from build123d import *

# Parameters (mm, degrees)
F0_W     = 149.5
F0_H     = 13
F0_R     = 3.1
F1_DEPTH = 18
F3_DEPTH = 10.25
F4_W     = 119.5
F4_H     = 7
F5_DEPTH = 18.001
F7_DEPTH = 25


with BuildPart() as f1:
    # F0 (on Top) → F1 (new body)
    with BuildSketch(Plane.XY):
        Rectangle(F0_W, F0_H)
        with Locations((-68.75, 0.5)):
            Circle(F0_R, mode=Mode.SUBTRACT)
        with Locations((68.75, 0.5)):
            Circle(F0_R, mode=Mode.SUBTRACT)
    extrude(amount=F1_DEPTH)

    # F2 (on Right) → F3 (cut, symmetric)
    with BuildSketch(Plane.YZ):
        Polygon((-6.5, 0), (8.5, 0), (-6.5, 15), align=None)
    extrude(amount=F3_DEPTH, both=True, mode=Mode.SUBTRACT)

    # F4 (on face) → F5 (cut, through all)
    with BuildSketch(Plane.XY.offset(18)):
        with Locations((0, 3)):
            Rectangle(F4_W, F4_H)
    extrude(amount=-F5_DEPTH, mode=Mode.SUBTRACT)

    # F6 (on face) → F7 (cut)
    with BuildSketch(Plane.XZ.offset(6.5)):
        Polygon((-51.359004, 10), (-59.75, 0), (-19.75, 0), (-28.140996, 10), align=None)
        Polygon((28.140996, 10), (19.75, 0), (59.75, 0), (51.359004, 10), align=None)
    extrude(amount=-F7_DEPTH, mode=Mode.SUBTRACT)


solid = f1.part
Geometry check sheet. Reference: the model listing, model coordinates, mm. A direction names the side the tool comes from. Coordinates: 2 decimals unless noted, no trailing zeros. Write each loop counter-clockwise with the first axis right and the second up, starting at its lowest first coordinate (ties: lowest second). Pieces come first, ordered by that corner, then holes. Notation, with made-up numbers: (-37, -37.75) -> (-32, -37.75) arc R36 cw to (-32, -3.75) -> close; hole circle Ø8 at (-12.5, -4.75). An arc over 180 degrees is marked (long way). One line per question, with ' | ' between items.
1. Draft check along X on faces 6 (the flat face through (74.75, 0, 9)), 7 (the flat face through (24.004, -3.542, 5.07)), 8 (the flat face through (-1, -6.5, 17)), 9 (the cylindrical face through (-65.793, 1.431, 8.874)). Enter one of: +X half, -X half, draft (parallel to the pull), parting line (faces both ways), or undercut.
Answers:
face 6: +X half | face 7: undercut | face 8: draft | face 9: undercut
2. Cross-section at D-D on x = 18. Record the cut outline in (y, z).
Answers:
outline: (-6.5, 0) -> (-0.5, 0) -> (-0.5, 18) -> (-6.5, 18) -> close
3. Cross-section at C-C on z = 6.25. Record the cut outline in (x, y), and give its area (3 significant figures).
Answers:
outline: (-74.75, -6.5) -> (-54.51, -6.5) -> (-54.51, -0.5) -> (-59.75, -0.5) -> (-59.75, 6.5) -> (-74.75, 6.5) -> close; (-24.99, -6.5) -> (-10.25, -6.5) -> (-10.25, -0.5) -> (-24.99, -0.5) -> close; (10.25, -6.5) -> (24.99, -6.5) -> (24.99, -0.5) -> (10.25, -0.5) -> close; (54.51, -6.5) -> (74.75, -6.5) -> (74.75, 6.5) -> (59.75, 6.5) -> (59.75, -0.5) -> (54.51, -0.5) -> close; hole circle Ø6.2 at (-68.75, 0.5); hole circle Ø6.2 at (68.75, 0.5) | area: 569 mm²
4. Depth check by flat-ended pin: pin 1 Ø3 at (x, y) = (39.5, -4.5) entering from -Z; pin 2 Ø8 at (x, z) = (-42, 7.5) entering from +Y. Enter the tip coordinate at first touch or a pass-through.
Answers:
pin 1: stops at z = 10 | pin 2: stops at y = -0.5
5. Cross-section at B-B on x = 68.75. Record the cut outline in (y, z), and give its area (3 significant figures).
Answers:
outline: (-6.5, 0) -> (-2.6, 0) -> (-2.6, 18) -> (-6.5, 18) -> close; (3.6, 0) -> (6.5, 0) -> (6.5, 18) -> (3.6, 18) -> close | area: 122 mm²
6. Cross-section at A-A on z = 16.5. Record the cut outline in (x, y).
Answers:
outline: (-74.75, -6.5) -> (74.75, -6.5) -> (74.75, 6.5) -> (59.75, 6.5) -> (59.75, -0.5) -> (-59.75, -0.5) -> (-59.75, 6.5) -> (-74.75, 6.5) -> close; hole circle Ø6.2 at (-68.75, 0.5); hole circle Ø6.2 at (68.75, 0.5)
7. Thickness scan on probe 1 along X at (y, z) = (0.75, 7.75); probe 2 along Y at (x, z) = (-68.75, 10.25); probe 3 along X at (y, z) = (-1.75, 12.25). Record the ranges inside material, lowest first. Write a range as from..to.
Answers:
probe 1: x = -74.75..-71.84, -65.66..-59.75, 59.75..65.66, 71.84..74.75 | probe 2: y = -6.5..-2.6, 3.6..6.5 | probe 3: x = -74.75..-70.88, -66.62..66.62, 70.88..74.75
8. Set-up check for faces 1 (the cylindrical face through (71.707, 1.431, 8.874)), 2 (the flat face through (-59.75, 3, 9)), 3 (the flat face through (-67, 6.5, 9)), 4 (the flat face through (-23.887, -3.542, 4.93)), 5 (the flat face through (0.1, -3.5, 12)): record each of +Z, -Z, +X, -X, +Y, -Y from which the full face is reachable in a straight line by a thin tool's end or side.
Answers:
face 1: +Z, -Z | face 2: +Z, -Z, +Y | face 3: +Z, -Z, +X, -X, +Y | face 4: -Z, +Y, -Y | face 5: -Z, -Y
